```python
from build123d import *

# Parameters (mm, degrees)
SKETCH1_W                    = 75
SKETCH1_H                    = 65
BASE_FLANGE1_DEPTH           = 0.81
EDGE_FLANGE1_STRIP_W         = 4.7132
EDGE_FLANGE1_STRIP_H         = 0.81
EDGE_FLANGE1_STRIP_CUT_DEPTH = 75
EDGE_FLANGE1_DEPTH           = 75
EDGE_FLANGE2_DEPTH           = 40.4534
EDGE_FLANGE2_BEND_DEPTH      = 40.4534
EDGE_FLANGE3_DEPTH           = 64.2634
EDGE_FLANGE3_BEND_DEPTH      = 64.2634
CUT_EXTRUDE1_REACH           = 113.546
CUT_EXTRUDE2_REACH           = 111.732
SKETCH24_R                   = 4
SKETCH24_R_2                 = 1.5
SKETCH24_R_3                 = 1.55
CUT_EXTRUDE3_REACH           = 111.732
SKETCH25_R                   = 2


# Sheet-metal steps are written as plain solids
with BuildPart() as part:
    # Sketch1 → Base-Flange1 (new body)
    with BuildSketch(Plane(origin=(0, 0, 0), x_dir=(1, 0, 0), z_dir=(0, 1, 0))):
        with Locations((37.5, 32.5)):
            Rectangle(SKETCH1_W, SKETCH1_H)
    extrude(amount=-BASE_FLANGE1_DEPTH)

    # Edge-Flange1 strip (across the edge) → Edge-Flange1 strip cut (cut)
    with BuildSketch(Plane(origin=(75, 0, -65), x_dir=(0, 0, 1), z_dir=(-1, 0, 0))):
        with Locations((-1.62, -0.405)):
            Rectangle(EDGE_FLANGE1_STRIP_W, EDGE_FLANGE1_STRIP_H)
    extrude(amount=EDGE_FLANGE1_STRIP_CUT_DEPTH, mode=Mode.SUBTRACT)

    # Edge-Flange1 section (across the edge) → Edge-Flange1 (add)
    with BuildSketch(Plane(origin=(75, 0, -65), x_dir=(0, 0, 1), z_dir=(-1, 0, 0))):
        with BuildLine():
            Line((-0.81, 0.7366), (-0.81, 41.19))
            Line((-0.81, 41.19), (0, 41.19))
            Line((0, 41.19), (0, 0.7366))
            ThreePointArc((0, 0.7366), (0.215745145, 0.215745145), (0.7366, 0))
            Line((0.7366, 0), (0.7366, -0.81))
            ThreePointArc((0.7366, -0.81), (-0.357011348, -0.357011348), (-0.81, 0.7366))
        make_face()
    extrude(amount=EDGE_FLANGE1_DEPTH)

    # Edge-Flange2 section (across the edge) → Edge-Flange2 (add)
    with BuildSketch(Plane(origin=(-1.7366, 41.19, -65), x_dir=(1, 0, 0), z_dir=(0, -1, 0))):
        with BuildLine():
            Line((-0.81, 0.7366), (-0.81, 42.19))
            Line((-0.81, 42.19), (0, 42.19))
            Line((0, 42.19), (0, 0.7366))
            ThreePointArc((0, 0.7366), (0.215745145, 0.215745145), (0.7366, 0))
            Line((0.7366, 0), (1.7366, 0))
            Line((1.7366, 0), (1.7366, -0.81))
            Line((1.7366, -0.81), (0.7366, -0.81))
            ThreePointArc((0.7366, -0.81), (-0.357011348, -0.357011348), (-0.81, 0.7366))
        make_face()
    extrude(amount=EDGE_FLANGE2_DEPTH)

    # Edge-Flange2 section 2 (across the edge) → Edge-Flange2 bend (add)
    with BuildSketch(Plane(origin=(76.7366, 0.7366, -65), x_dir=(-1, 0, 0), z_dir=(0, 1, 0))):
        with BuildLine():
            Line((-0.81, 0.7366), (-0.81, 42.19))
            Line((-0.81, 42.19), (0, 42.19))
            Line((0, 42.19), (0, 0.7366))
            ThreePointArc((0, 0.7366), (0.215745145, 0.215745145), (0.7366, 0))
            Line((0.7366, 0), (1.7366, 0))
            Line((1.7366, 0), (1.7366, -0.81))
            Line((1.7366, -0.81), (0.7366, -0.81))
            ThreePointArc((0.7366, -0.81), (-0.357011348, -0.357011348), (-0.81, 0.7366))
        make_face()
    extrude(amount=EDGE_FLANGE2_BEND_DEPTH)

    # Edge-Flange3 section (across the edge) → Edge-Flange3 (add)
    with BuildSketch(Plane(origin=(-0.7366, 0, -64.2634), x_dir=(1, 0, 0), z_dir=(0, 0, 1))):
        with BuildLine():
            Line((-0.81, 0.7366), (-0.81, 41.19))
            Line((-0.81, 41.19), (0, 41.19))
            Line((0, 41.19), (0, 0.7366))
            ThreePointArc((0, 0.7366), (0.215745145, 0.215745145), (0.7366, 0))
            Line((0.7366, 0), (0.7366, -0.81))
            ThreePointArc((0.7366, -0.81), (-0.357011348, -0.357011348), (-0.81, 0.7366))
        make_face()
    extrude(amount=EDGE_FLANGE3_DEPTH)

    # Edge-Flange3 section 2 (across the edge) → Edge-Flange3 bend (add)
    with BuildSketch(Plane(origin=(75.7366, 0, 0), x_dir=(-1, 0, 0), z_dir=(0, 0, -1))):
        with BuildLine():
            Line((-0.81, 0.7366), (-0.81, 41.19))
            Line((-0.81, 41.19), (0, 41.19))
            Line((0, 41.19), (0, 0.7366))
            ThreePointArc((0, 0.7366), (0.215745145, 0.215745145), (0.7366, 0))
            Line((0.7366, 0), (0.7366, -0.81))
            ThreePointArc((0.7366, -0.81), (-0.357011348, -0.357011348), (-0.81, 0.7366))
        make_face()
    extrude(amount=EDGE_FLANGE3_BEND_DEPTH)

    # Cut-Extrude1: up to this face of the body (flat: up to its plane)
    cut_extrude1_end = Plane(part.part.faces().sort_by_distance((77.5466, 20.9633, -43.5367))[0])
    # Sketch23 → Cut-Extrude1 (cut, up to the picked face)
    with BuildSketch(Plane.ZY.offset(2.5466), mode=Mode.PRIVATE) as cut_extrude1_sk1:
        Polygon((-64.2634, 41.19), (-22.81, 0.7366), (0, 0.7366), (0, 41.19), align=None)
    cut_extrude1_tool1 = split(extrude(cut_extrude1_sk1.sketch, amount=-CUT_EXTRUDE1_REACH, mode=Mode.PRIVATE), bisect_by=cut_extrude1_end, keep=Keep.BOTH, mode=Mode.PRIVATE)
    add(cut_extrude1_tool1.solids().sort_by(Axis((-2.5466, 24.173103, -23.412925), (1, 0, 0)))[0], mode=Mode.SUBTRACT)

    # Sketch24 → Cut-Extrude2 (cut, up to next)
    with BuildSketch(Plane(origin=(0, 0, -65.81), x_dir=(-1, 0, 0), z_dir=(0, 0, -1)), mode=Mode.PRIVATE) as cut_extrude2_sk1:
        with Locations(Location((-42.01805, 23.62082, 0), (0, 0, 90))):
            Circle(SKETCH24_R)
    cut_extrude2_tool1 = extrude(cut_extrude2_sk1.sketch, amount=-CUT_EXTRUDE2_REACH, mode=Mode.PRIVATE) & part.part
    # Sketch24 → Cut-Extrude2 (cut, up to next)
    with BuildSketch(Plane(origin=(0, 0, -65.81), x_dir=(-1, 0, 0), z_dir=(0, 0, -1)), mode=Mode.PRIVATE) as cut_extrude2_sk2:
        with Locations(Location((-42.01805, 33.83162, 0), (0, 0, 90))):
            Circle(SKETCH24_R_2)
    cut_extrude2_tool2 = extrude(cut_extrude2_sk2.sketch, amount=-CUT_EXTRUDE2_REACH, mode=Mode.PRIVATE) & part.part
    # Sketch24 → Cut-Extrude2 (cut, up to next)
    with BuildSketch(Plane(origin=(0, 0, -65.81), x_dir=(-1, 0, 0), z_dir=(0, 0, -1)), mode=Mode.PRIVATE) as cut_extrude2_sk3:
        with Locations(Location((-64.19225, 23.62082, 0), (0, 0, 90))):
            Circle(SKETCH24_R_2)
    cut_extrude2_tool3 = extrude(cut_extrude2_sk3.sketch, amount=-CUT_EXTRUDE2_REACH, mode=Mode.PRIVATE) & part.part
    # Sketch24 → Cut-Extrude2 (cut, up to next)
    with BuildSketch(Plane(origin=(0, 0, -65.81), x_dir=(-1, 0, 0), z_dir=(0, 0, -1)), mode=Mode.PRIVATE) as cut_extrude2_sk4:
        with Locations(Location((-42.01805, 13.41002, 0), (0, 0, 90))):
            Circle(SKETCH24_R_2)
    cut_extrude2_tool4 = extrude(cut_extrude2_sk4.sketch, amount=-CUT_EXTRUDE2_REACH, mode=Mode.PRIVATE) & part.part
    # Sketch24 → Cut-Extrude2 (cut, up to next)
    with BuildSketch(Plane(origin=(0, 0, -65.81), x_dir=(-1, 0, 0), z_dir=(0, 0, -1)), mode=Mode.PRIVATE) as cut_extrude2_sk5:
        with Locations(Location((-18.720201976, 5, 0), (0, 0, 90))):
            Circle(SKETCH24_R_3)
    cut_extrude2_tool5 = extrude(cut_extrude2_sk5.sketch, amount=-CUT_EXTRUDE2_REACH, mode=Mode.PRIVATE) & part.part
    # Sketch24 → Cut-Extrude2 (cut, up to next)
    with BuildSketch(Plane(origin=(0, 0, -65.81), x_dir=(-1, 0, 0), z_dir=(0, 0, -1)), mode=Mode.PRIVATE) as cut_extrude2_sk6:
        with Locations(Location((-56.279798024, 5, 0), (0, 0, 270))):
            Circle(SKETCH24_R_3)
    cut_extrude2_tool6 = extrude(cut_extrude2_sk6.sketch, amount=-CUT_EXTRUDE2_REACH, mode=Mode.PRIVATE) & part.part
    # Sketch24 → Cut-Extrude2 (cut, up to next)
    with BuildSketch(Plane(origin=(0, 0, -65.81), x_dir=(-1, 0, 0), z_dir=(0, 0, -1)), mode=Mode.PRIVATE) as cut_extrude2_sk7:
        with Locations(Location((-32.98195, 13.41002, 0), (0, 0, 270))):
            Circle(SKETCH24_R_2)
    cut_extrude2_tool7 = extrude(cut_extrude2_sk7.sketch, amount=-CUT_EXTRUDE2_REACH, mode=Mode.PRIVATE) & part.part
    # Sketch24 → Cut-Extrude2 (cut, up to next)
    with BuildSketch(Plane(origin=(0, 0, -65.81), x_dir=(-1, 0, 0), z_dir=(0, 0, -1)), mode=Mode.PRIVATE) as cut_extrude2_sk8:
        with Locations(Location((-10.80775, 23.62082, 0), (0, 0, 270))):
            Circle(SKETCH24_R_2)
    cut_extrude2_tool8 = extrude(cut_extrude2_sk8.sketch, amount=-CUT_EXTRUDE2_REACH, mode=Mode.PRIVATE) & part.part
    # Sketch24 → Cut-Extrude2 (cut, up to next)
    with BuildSketch(Plane(origin=(0, 0, -65.81), x_dir=(-1, 0, 0), z_dir=(0, 0, -1)), mode=Mode.PRIVATE) as cut_extrude2_sk9:
        with Locations(Location((-32.98195, 33.83162, 0), (0, 0, 270))):
            Circle(SKETCH24_R_2)
    cut_extrude2_tool9 = extrude(cut_extrude2_sk9.sketch, amount=-CUT_EXTRUDE2_REACH, mode=Mode.PRIVATE) & part.part
    # Sketch24 → Cut-Extrude2 (cut, up to next)
    with BuildSketch(Plane(origin=(0, 0, -65.81), x_dir=(-1, 0, 0), z_dir=(0, 0, -1)), mode=Mode.PRIVATE) as cut_extrude2_sk10:
        with Locations(Location((-32.98195, 23.62082, 0), (0, 0, 270))):
            Circle(SKETCH24_R)
    cut_extrude2_tool10 = extrude(cut_extrude2_sk10.sketch, amount=-CUT_EXTRUDE2_REACH, mode=Mode.PRIVATE) & part.part
    add(cut_extrude2_tool1.solids().sort_by_distance((42.01805, 23.62082, -65.81))[0], mode=Mode.SUBTRACT)
    add(cut_extrude2_tool2.solids().sort_by_distance((42.01805, 33.83162, -65.81))[0], mode=Mode.SUBTRACT)
    add(cut_extrude2_tool3.solids().sort_by_distance((64.19225, 23.62082, -65.81))[0], mode=Mode.SUBTRACT)
    add(cut_extrude2_tool4.solids().sort_by_distance((42.01805, 13.41002, -65.81))[0], mode=Mode.SUBTRACT)
    add(cut_extrude2_tool5.solids().sort_by_distance((18.720202, 5, -65.81))[0], mode=Mode.SUBTRACT)
    add(cut_extrude2_tool6.solids().sort_by_distance((56.279798, 5, -65.81))[0], mode=Mode.SUBTRACT)
    add(cut_extrude2_tool7.solids().sort_by_distance((32.98195, 13.41002, -65.81))[0], mode=Mode.SUBTRACT)
    add(cut_extrude2_tool8.solids().sort_by_distance((10.80775, 23.62082, -65.81))[0], mode=Mode.SUBTRACT)
    add(cut_extrude2_tool9.solids().sort_by_distance((32.98195, 33.83162, -65.81))[0], mode=Mode.SUBTRACT)
    add(cut_extrude2_tool10.solids().sort_by_distance((32.98195, 23.62082, -65.81))[0], mode=Mode.SUBTRACT)

    # Sketch25 → Cut-Extrude3 (cut, up to next)
    with BuildSketch(Plane(origin=(0, 0, 0), x_dir=(1, 0, 0), z_dir=(0, 1, 0)), mode=Mode.PRIVATE) as cut_extrude3_sk1:
        with Locations(Location((62.5, 16.75, 0), (0, 0, 270))):
            Circle(SKETCH25_R)
    cut_extrude3_tool1 = extrude(cut_extrude3_sk1.sketch, amount=-CUT_EXTRUDE3_REACH, mode=Mode.PRIVATE) & part.part
    # Sketch25 → Cut-Extrude3 (cut, up to next)
    with BuildSketch(Plane(origin=(0, 0, 0), x_dir=(1, 0, 0), z_dir=(0, 1, 0)), mode=Mode.PRIVATE) as cut_extrude3_sk2:
        with Locations(Location((12.5, 16.75, 0), (0, 0, 270))):
            Circle(SKETCH25_R)
    cut_extrude3_tool2 = extrude(cut_extrude3_sk2.sketch, amount=-CUT_EXTRUDE3_REACH, mode=Mode.PRIVATE) & part.part
    add(cut_extrude3_tool1.solids().sort_by_distance((62.5, 0, -16.75))[0], mode=Mode.SUBTRACT)
    add(cut_extrude3_tool2.solids().sort_by_distance((12.5, 0, -16.75))[0], mode=Mode.SUBTRACT)


solid = part.part
```
Can you work these out from the model? Positions are in its coordinate system, mm. A direction names the side the tool comes from. Coordinates: 2 decimals unless noted, no trailing zeros. Loops run counter-clockwise (first coordinate to the right, second up) from the corner with the lowest first, then second, coordinate; pieces in that order, holes last. Notation, with made-up numbers: (-38.5, 48) -> (7.5, 48) arc R26 cw to (7.5, 73) -> close; hole circle Ø4 at (71.25, -24.75). An arc over 180 degrees is marked (long way). Answer as a JSON object with one key per item and string values.
1) For faces 1 (the face through (37, 0, -33)), 2 (the face through (76.547, 12, -52)), 3 (the face through (62.86, 24.31, -65.41)), which set-ups out of +Z, -Z, +X, -X, +Y, -Y let a thin tool reach every point of the face, with its end or its side?
Results:
{"face 1": "+Z, +Y", "face 2": "+Z, +Y, -Y", "face 3": "+Z, -Z"}
2) Imagine slicing it at B-B (x = 53.5). Please give me the cut outline in (y, z), then the cut area to 3 significant figures.
Results:
{"outline": "(-0.81, -64.26) arc R1.55 ccw to (0.74, -65.81) -> (41.19, -65.81) -> (41.19, -65) -> (0.74, -65) arc R0.74 cw to (0, -64.26) -> (0, 0) -> (-0.81, 0) -> close", "area": "86.3 mm^2"}
3) Imagine slicing it at C-C (y = 5). Please give me the cut outline in (x, z).
Results:
{"outline": "(-2.55, -64.26) arc R1.55 ccw to (-1, -65.81) -> (17.17, -65.81) -> (17.17, -65) -> (-1, -65) arc R0.74 cw to (-1.74, -64.26) -> (-1.74, -27.18) -> (-2.55, -27.18) -> close; (-1.55, -64.26) -> (-0.74, -64.26) -> (-0.74, -27.18) -> (-1.55, -27.18) -> close; (20.27, -65.81) -> (54.73, -65.81) -> (54.73, -65) -> (20.27, -65) -> close; (57.83, -65.81) -> (76, -65.81) arc R1.55 ccw to (77.55, -64.26) -> (77.55, -27.18) -> (76.74, -27.18) -> (76.74, -64.26) arc R0.74 cw to (76, -65) -> (57.83, -65) -> close; (75.74, -64.26) -> (76.55, -64.26) -> (76.55, -27.18) -> (75.74, -27.18) -> close"}
4) If I drill on line 1 (X direction, y = 2.5, z = -58.5); line 2 (X direction, y = 5, z = -65.6); line 3 (Y direction, x = 63, z = -4), over which ranges is the centre line in solid material (lowest first)?
Results:
{"line 1": "x = -2.55 to -1.74, -1.55 to -0.74, 75.74 to 76.55, 76.74 to 77.55", "line 2": "x = -1.78 to 17.17, 20.27 to 54.73, 57.83 to 76.78", "line 3": "y = -0.81 to 0"}
5) Imagine slicing it at D-D (y = 26.5). Please give me the cut outline in (x, z), then the cut area to 3 significant figures.
Results:
{"outline": "(-2.55, -64.26) arc R1.55 ccw to (-1, -65.81) -> (30.21, -65.81) -> (30.21, -65) -> (-1, -65) arc R0.74 cw to (-1.74, -64.26) -> (-1.74, -49.21) -> (-2.55, -49.21) -> close; (-1.55, -64.26) -> (-0.74, -64.26) -> (-0.74, -49.21) -> (-1.55, -49.21) -> close; (35.76, -65.81) -> (39.24, -65.81) -> (39.24, -65) -> (35.76, -65) -> close; (44.79, -65.81) -> (76, -65.81) arc R1.55 ccw to (77.55, -64.26) -> (77.55, -49.21) -> (76.74, -49.21) -> (76.74, -64.26) arc R0.74 cw to (76, -65) -> (44.79, -65) -> close; (75.74, -64.26) -> (76.55, -64.26) -> (76.55, -49.21) -> (75.74, -49.21) -> close", "area": "105 mm^2"}
6) For P1, Ø5, axis at x = 21, y = 36.5, coming from the +Z side; P2, Ø2.5, axis at x = 18.72, y = 5, coming from the -Z side; P3, Ø0.9, axis at x = 76, z = -15, coming from the +Y side; P4, Ø0.8, axis at y = 0.5, z = -65, coming from the +X side, each with a flat end and sliding along its axis, tell me the tip position at first contact or that it passes through.
Results:
{"P1": "stops at z = -65", "P2": "passes through", "P3": "stops at y = 0.74", "P4": "stops at x = 77.49"}
7) Thinking about a two-plate mould opening in Z: for faces 4 (the face through (37, 21, -65.81)), 5 (the face through (77, 0.737, -44)), 6 (the face through (76.14, 21.25, -43.83)), 7 (the face through (64.2, -0.4, -15.7)), which applies, pulls with the +Z half, pulls with the -Z half, needs draft (parallel to the pull), parting line crosses it, or undercut?
Results:
{"face 4": "pulls with the -Z half", "face 5": "needs draft", "face 6": "pulls with the +Z half", "face 7": "undercut"}
8) Imagine slicing it at A-A (z = -16.75). Please give me the cut outline in (x, y).
Results:
{"outline": "(-1.55, 0.74) arc R1.55 ccw to (0, -0.81) -> (10.5, -0.81) -> (10.5, 0) -> (0, 0) arc R0.74 cw to (-0.74, 0.74) -> close; (14.5, -0.81) -> (60.5, -0.81) -> (60.5, 0) -> (14.5, 0) -> close; (64.5, -0.81) -> (75, -0.81) arc R1.55 ccw to (76.55, 0.74) -> (75.74, 0.74) arc R0.74 cw to (75, 0) -> (64.5, 0) -> close"}
